from build123d import *
from OCP.BRepFilletAPI import BRepFilletAPI_MakeChamfer

# Parameters (mm, degrees)
SKETCH_1_R          = 2.5
EXTRUDE_1_DEPTH     = 15
SKETCH_2_R          = 2.5
SKETCH_2_R_2        = 2
CUT_EXTRUDE_1_DEPTH = 0.8
CHAMFER_1_SIZE      = 0.5
CHAMFER_1_SIZE2     = 0.419549816


with BuildPart() as part:
    # 草图1 → 凸台-拉伸1 (new body)
    with BuildSketch(Plane(origin=(0, 0, 0), x_dir=(1, 0, 0), z_dir=(0, 1, 0))):
        with Locations(Location((0, 0, 0), (0, 0, 270))):
            Circle(SKETCH_1_R)
    extrude_1 = extrude(amount=EXTRUDE_1_DEPTH)

    # 草图2 → 切除-拉伸1 (cut)
    with BuildSketch(Plane(origin=(0, 12.5, 0), x_dir=(-1, 0, 0), z_dir=(0, -1, 0))):
        with Locations(Location((0, 0, 0), (0, 0, 90))):
            Circle(SKETCH_2_R)
        with Locations(Location((0, 0, 0), (0, 0, 90))):
            Circle(SKETCH_2_R_2, mode=Mode.SUBTRACT)
    cut_extrude_1 = extrude(amount=-CUT_EXTRUDE_1_DEPTH, mode=Mode.SUBTRACT)

    # 镜向1: 凸台-拉伸1, 切除-拉伸1 across plane
    add(extrude_1.mirror(Plane.ZX))
    add(cut_extrude_1.mirror(Plane.ZX), mode=Mode.SUBTRACT)

    # 倒角1: one chamfer whose edges measure the first distance from different faces: ONE call of the kernel's chamfer builder (chamfer() names one face for all edges)
    chamfer_1_edges_1 = [part.edges().sort_by_distance(p)[0] for p in [
        (0, -15, -2.5),
    ]]
    chamfer_1_side_1 = [part.faces().sort_by_distance(p)[0] for p in [
        (0, -15, 0),
    ]]
    chamfer_1_edges_2 = [part.edges().sort_by_distance(p)[0] for p in [
        (0, 15, -2.5),
    ]]
    chamfer_1_side_2 = [part.faces().sort_by_distance(p)[0] for p in [
        (0, 14.15, -2.5),
    ]]
    chamfer_1 = BRepFilletAPI_MakeChamfer(part.part.solid().wrapped)
    for e in chamfer_1_edges_1:
        chamfer_1.Add(CHAMFER_1_SIZE, CHAMFER_1_SIZE2, e.wrapped, chamfer_1_side_1[0].wrapped)  # the first distance lies on this face
    for e in chamfer_1_edges_2:
        chamfer_1.Add(CHAMFER_1_SIZE, CHAMFER_1_SIZE2, e.wrapped, chamfer_1_side_2[0].wrapped)  # the first distance lies on this face
    add(Compound.cast(chamfer_1.Shape()), mode=Mode.REPLACE)


solid = part.part
Geometry: final body of the model. Coordinates: model frame, mm. A direction names the side the tool comes from. Coordinates: 2 decimals unless noted, no trailing zeros. Order: outer loops, then holes, each group sorted by start corner. A loop starts at its lowest first (then second) coordinate and runs counter-clockwise, first axis right, second up.
(1) Draft query along Y for faces 3 (the face through (0, -15, 0)), 4 (the face through (2, 13.3, 1)), 5 (the face through (-2.44, -13.93, -0.54)). Return one class per face: pulls with the +Y half, pulls with the -Y half, needs draft (parallel to the pull), parting line crosses it, or undercut.
(2) Access query for faces 1 (the face through (-2, 13, 0)), 2 (the face through (-2.44, 13.89, -0.54)). Directions: +Z, -Z, +X, -X, +Y, -Y. A direction counts if a zero-diameter tool reaches every point of the face in a straight line with its end or side. Return the directions, or none.
(3) Section query B-B (y = -3). Return the cut outline in (x, z), plus the area to 3 significant figures.
(4) Material intervals for probe 1 along Y at (x, z) = (-1.8, -1.65); probe 2 along Y at (x, z) = (2.15, 0); probe 3 along Z at (x, y) = (0.1, 3.75), sorted ascending.
(5) Section query A-A (y = -12.75). Return the cut outline in (x, z).
Solution:
1. face 3: pulls with the -Y half
1. face 4: undercut
1. face 5: needs draft
2. face 1: none
2. face 2: +Y, -Y
3. outline: circle Ø5 at (0, 0)
3. area: 19.6 mm2
4. probe 1: y = -14.63 to -13.3, -12.5 to 12.5, 13.3 to 14.57
4. probe 2: y = -14.87 to -13.3, -12.5 to 12.5, 13.3 to 14.92
4. probe 3: z = -2.5 to 2.5
5. outline: circle Ø4 at (0, 0)
